Job drawing, mm, ordinate dimensions from the low corner. One solid piece. Round coordinates to 2 decimals unless told otherwise and drop trailing zeros. Loops run counter-clockwise (first coordinate to the right, second up) from the corner with the lowest first, then second, coordinate; pieces in that order, holes last. Notation, with made-up numbers: M -33.5,-25 L 25.5,-25 A16 ccw 25.5,-11 Z; hole C 76,4.5 d2. An arc over 180 degrees is marked long. One line per item, written item: value.
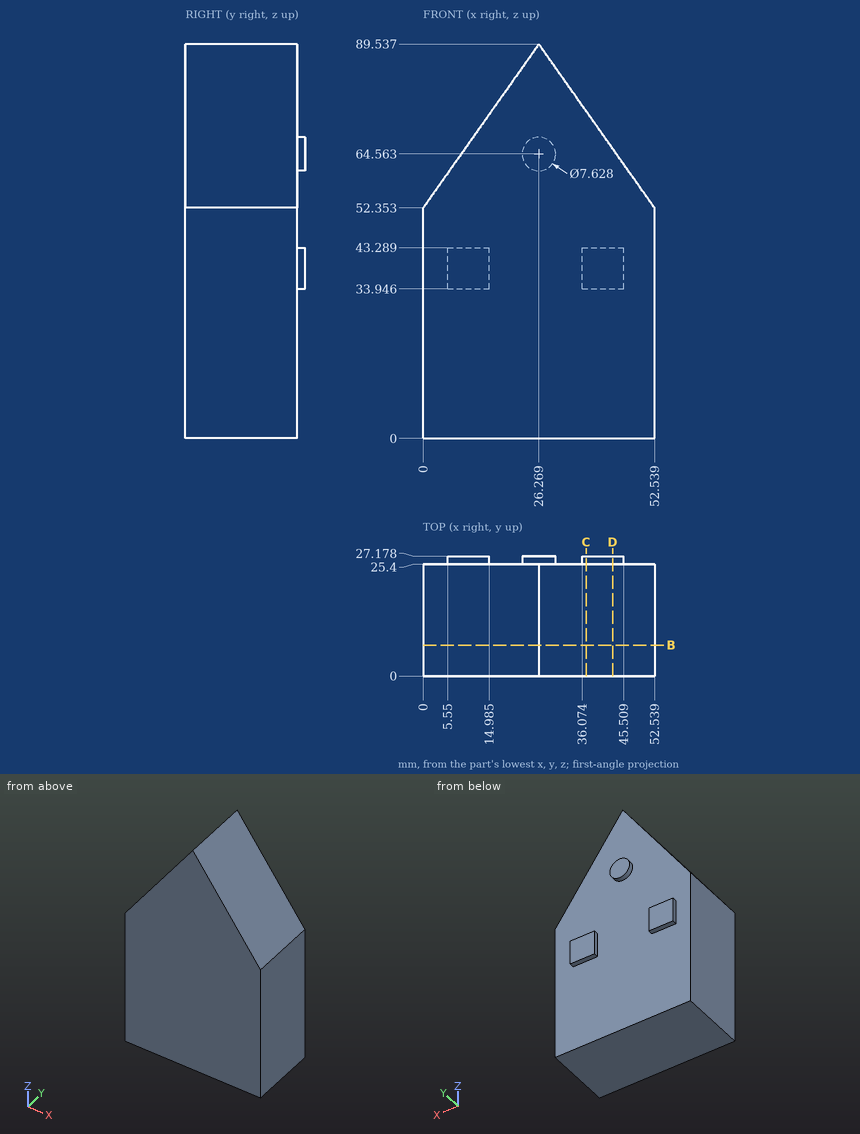
Item 1: Slice it at B-B, the plane y = 7. Give the cut face in (x, z).
Check values:
outline: M 0,0 L 52.54,0 L 52.54,52.35 L 26.27,89.54 L 0,52.35 Z
Item 2: Slice it at D-D, the plane x = 43. Give the cut face in (y, z) (1 decimal).
Check values:
outline: M 0,0 L 25.4,0 L 25.4,33.9 L 27.2,33.9 L 27.2,43.3 L 25.4,43.3 L 25.4,65.9 L 0,65.9 Z
Item 3: Wall check: line 1 along Y through (x, z) = (15.5, 71.5); line 2 along Z through (x, y) = (4.5, 20.75) (1 decimal); line 3 along X through (y, z) = (12.75, 71) (1 decimal). Give the ranges that are in metal, low to high.
Check values:
line 1: y = 0 to 25.4
line 2: z = 0 to 58.7
line 3: x = 13.2 to 39.4
Item 4: Slice it at C-C, the plane x = 37. Give the cut face in (y, z), and give its area (4 significant figures).
Check values:
outline: M 0,0 L 25.4,0 L 25.4,33.95 L 27.18,33.95 L 27.18,43.29 L 25.4,43.29 L 25.4,74.35 L 0,74.35 Z
area: 1,905 mm2
Item 5: Drop flat-ended pins along their axis: P1, Ø5, axis at x = 24, z = 46, coming from the +Y side; P2, Ø0.5, axis at x = 41, y = 26.5, coming from the +Z side; P3, Ø0.5, axis at y = 26, z = 40.5, coming from the -X side; P4, Ø2, axis at y = 26, z = 41, coming from the +X side. Give the stop position or say it passes through.
Check values:
P1: stops at y = 25.4
P2: stops at z = 43.29
P3: stops at x = 5.55
P4: stops at x = 52.54
